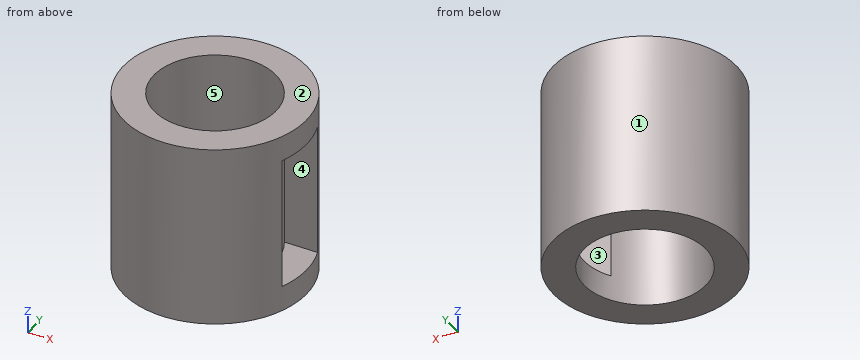
Solid Edge part; units mm, degrees
sketch "Sketch1" plane through (0, 0, 0) normal (0, 0, 1) x (1, 0, 0)
  circle A0 centre (0, 0) radius 6
  circle A1 centre (0, 0) radius 9
extrude "Protrusion1" add sketch "Sketch1" along normal blind 18
sketch "Sketch2" plane through (0, 0, 0) normal (-1, 0, 0) x (0, -1, 0)
  line L0 (-3.1, 15.5) -> (3.1, 15.5)
  line L1 (3.1, 15.5) -> (3.1, 2.5)
  line L2 (3.1, 2.5) -> (-3.1, 2.5)
  line L3 (-3.1, 2.5) -> (-3.1, 15.5)
  dimension "D1" = 3.1
  dimension "D2" = 3.1
extrude "Cutout1" cut sketch "Sketch2" against normal up to next
Here's how the part is built. I have some questions about the finished solid (model axes, mm). Face numbers are marked on the shaded views. A direction names the side the tool comes from. Round coordinates to 2 decimals unless told otherwise and drop trailing zeros. Write each loop counter-clockwise with the first axis right and the second up, starting at its lowest first coordinate (ties: lowest second). Pieces come first, ordered by that corner, then holes. Notation, with made-up numbers: (-24, 51.5) -> (-6, 51.5) arc R13 ccw to (-6, 76.5) -> close; hole circle Ø2 at (8.25, 69.25). An arc over 180 degrees is marked (long way). One line per item, written item: value.
1) Suppose I cut it at B-B on x = 0. List the corners of the cut face in (y, z) for me, plus the area to 3 significant figures.
Filled sheet:
outline: (-9, 0) -> (-6, 0) -> (-6, 18) -> (-9, 18) -> close; (6, 0) -> (9, 0) -> (9, 18) -> (6, 18) -> close
area: 108 mm2
2) Suppose I cut it at D-D on z = 5. List the corners of the cut face in (x, y) for me, plus the area to 3 significant figures.
Filled sheet:
outline: (5.14, -3.1) arc R6 cw (long way) to (5.14, 3.1) -> (8.45, 3.1) arc R9 ccw (long way) to (8.45, -3.1) -> close
area: 122 mm2
3) We'd pull the mould along Y, two halves only. Please class the marked faces 1, 2 and 3: released by +Y, released by -Y, zero draft, split by the parting line, or undercut.
Filled sheet:
face 1: split by the parting line
face 2: zero draft
face 3: undercut
4) If I drill on line 1 (Y direction, x = 0, z = 8.5); line 2 (Z direction, x = 8, y = 2.25); line 3 (Y direction, x = 5.5, z = 3.5), over which ranges is the centre line in solid material (lowest first)? Write a range as [from, to].
Filled sheet:
line 1: y = [-9, -6], [6, 9]
line 2: z = [0, 2.5], [15.5, 18]
line 3: y = [-7.12, -3.1], [3.1, 7.12]
5) For the marked faces 4 and 5, which set-ups out of +Z, -Z, +X, -X, +Y, -Y let a thin tool reach every point of the face, with its end or its side?
Filled sheet:
face 4: +X
face 5: +Z, -Z
6) I'm going to push flat-ended pins straight in: pin 1 Ø3.5 at (x, z) = (7, 8.5) entering from +Y; pin 2 Ø6 at (x, y) = (4.5, -0.5) entering from +Z; pin 3 Ø5 at (y, z) = (-2.5, 14) entering from +X; pin 4 Ø1 at (x, z) = (4.5, 6.5) entering from -Y. Where does each tip first touch, or does it pass through?
Filled sheet:
pin 1: stops at y = 7.31
pin 2: stops at z = 18
pin 3: stops at x = 8.99
pin 4: stops at y = -8.06
7) Suppose I cut it at C-C on y = 5. List the corners of the cut face in (x, z) for me, plus the area to 3 significant figures.
Filled sheet:
outline: (-7.48, 0) -> (-3.32, 0) -> (-3.32, 18) -> (-7.48, 18) -> close; (3.32, 0) -> (7.48, 0) -> (7.48, 18) -> (3.32, 18) -> close
area: 150 mm2
8) Suppose I cut it at A-A on y = 0. List the corners of the cut face in (x, z) for me, plus the area to 3 significant figures.
Filled sheet:
outline: (-9, 0) -> (-6, 0) -> (-6, 18) -> (-9, 18) -> close; (6, 0) -> (9, 0) -> (9, 2.5) -> (6, 2.5) -> close; (6, 15.5) -> (9, 15.5) -> (9, 18) -> (6, 18) -> close
area: 69.0 mm2
